For this review, use the dimensioned drawing (mm, ordinates from the lowest corner) and the shaded views. A direction names the side the tool comes from. Round coordinates to 2 decimals unless told otherwise and drop trailing zeros. Write each loop counter-clockwise with the first axis right and the second up, starting at its lowest first coordinate (ties: lowest second). Pieces come first, ordered by that corner, then holes. Notation, with made-up numbers: M -39,63.25 L -22,63.25 A28 ccw -22,97.25 Z; hole C 4.25,-11.5 d2. An arc over 180 degrees is marked long. Use one line per item in the form item = value. Start each with the question number.
Item 1: Add section D-D (x = 61). State the section outline as (y, z) points, and give its area (3 significant figures).
Item 2: Add section C-C (y = 15). State the section outline as (x, z) points.
Item 3: For P1, Ø4, axis at y = 23, z = 149, coming from the +X side; P2, Ø4, axis at x = 47, y = 39.5, coming from the +Z side; P3, Ø2, axis at x = 166.5, z = 101.5, coming from the +Y side, all flat-tipped, find the tip position at first contact; note any pin that passes through.
Item 4: Add section B-B (z = 82). State the section outline as (x, y) points, and give its area (4 significant figures).
Item 5: For the marked faces 1 and 2, list the 3-axis set-ups (+Z, -Z, +X, -X, +Y, -Y) from which the entire face can be reached by the end or side of a thin tool; tool diameter is ignored.
Item 6: For line 1 (X direction, y = 38.25, z = 82); line 2 (Z direction, x = 95.5, y = 13.5); line 3 (Y direction, x = 126.5, z = 79), list the stretches that pass through material, from the lowest coordinate up. Write a range as [from, to].
Item 7: Add section A-A (x = 175). State the section outline as (y, z) points.
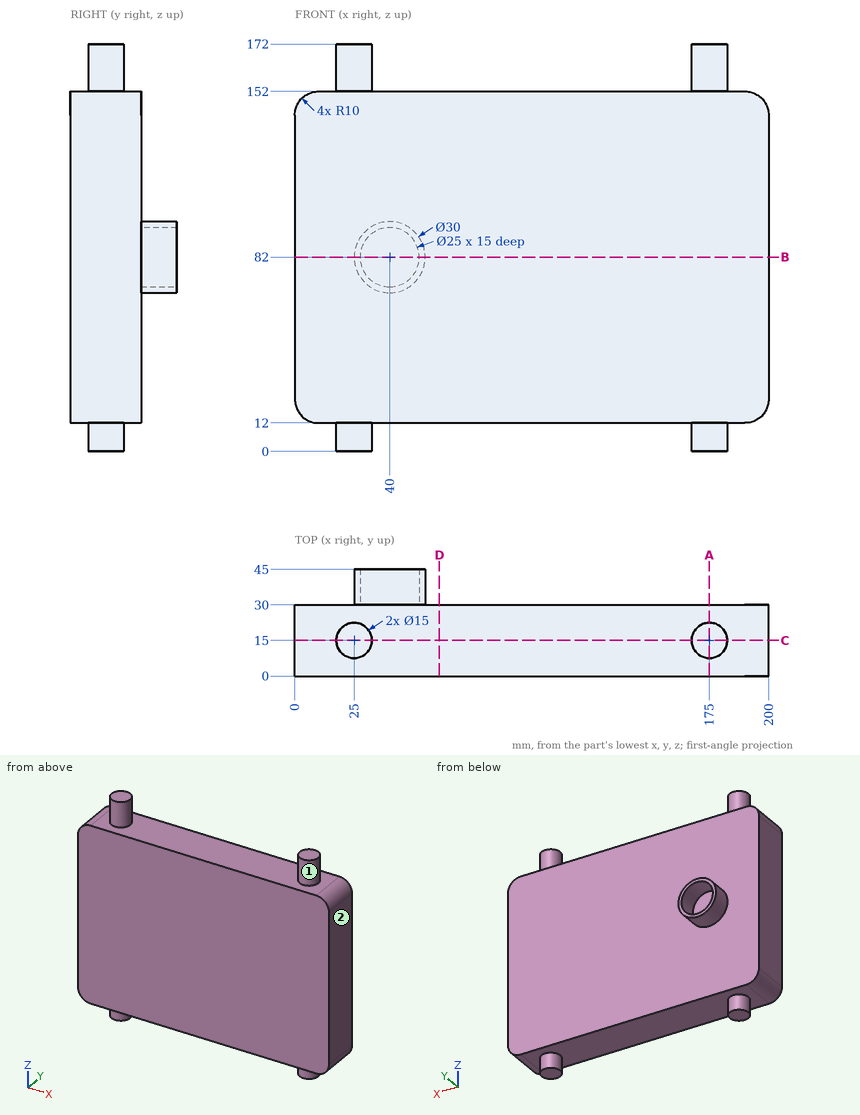
Calculated:
q1.outline = M 0,12 L 30,12 L 30,152 L 0,152 Z
q1.area = 4,200 mm^2
q2.outline = M 0,22 A10 ccw 10,12 L 17.5,12 L 17.5,0 L 32.5,0 L 32.5,12 L 167.5,12 L 167.5,0 L 182.5,0 L 182.5,12 L 190,12 A10 ccw 200,22 L 200,142 A10 ccw 190,152 L 182.5,152 L 182.5,172 L 167.5,172 L 167.5,152 L 32.5,152 L 32.5,172 L 17.5,172 L 17.5,152 L 10,152 A10 ccw 0,142 Z
q3.P1 = 198.66
q3.P2 = 96.14
q3.P3 = 30
q4.outline = M 0,0 L 200,0 L 200,30 L 55,30 L 55,45 L 52.5,45 L 52.5,30 L 27.5,30 L 27.5,45 L 25,45 L 25,30 L 0,30 Z
q4.area = 6,075 mm^2
q5.face_1 = +Z
q5.face_2 = +Z, -Z, +X, +Y, -Y
q6.line_1 = [25, 27.5], [52.5, 55]
q6.line_2 = [12, 152]
q6.line_3 = [0, 30]
q7.outline = M 0,12 L 7.5,12 L 7.5,0 L 22.5,0 L 22.5,12 L 30,12 L 30,152 L 22.5,152 L 22.5,172 L 7.5,172 L 7.5,152 L 0,152 Z
